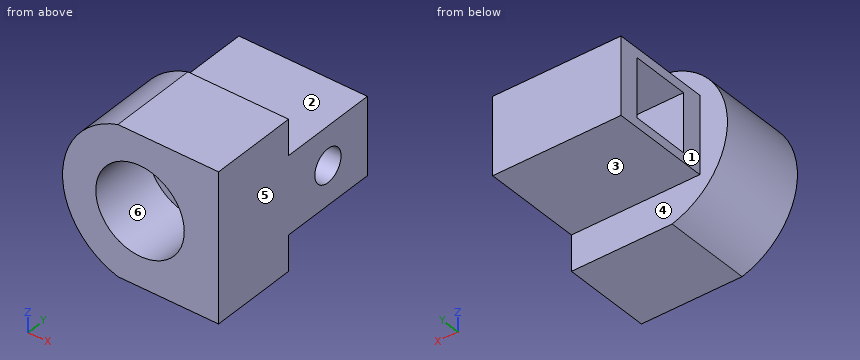
from build123d import *

# Parameters (mm, degrees)
SKETCH1_R           = 7
SKETCH1_R_2         = 4
BOSS_EXTRUDE1_DEPTH = 6
SKETCH2_R           = 7
BOSS_EXTRUDE2_DEPTH = 10
CUT_EXTRUDE1_DEPTH  = 8
SKETCH4_W           = 4.3
SKETCH4_H           = 6.3
CUT_EXTRUDE2_DEPTH  = 6
SKETCH5_OUTSIDE_W   = 21.092
SKETCH5_OUTSIDE_H   = 21.092
CUT_EXTRUDE3_DEPTH  = 8
BOSS_EXTRUDE3_DEPTH = 8
SKETCH9_R           = 7
CUT_EXTRUDE6_DEPTH  = 8
SKETCH10_W          = 9
SKETCH10_H          = 7
BOSS_EXTRUDE5_DEPTH = 9
SKETCH11_W          = 5.3
SKETCH11_H          = 5.3
CUT_EXTRUDE7_DEPTH  = 6
BOSS_EXTRUDE6_DEPTH = 8
SKETCH14_W          = 7
SKETCH14_H          = 9
BOSS_EXTRUDE7_DEPTH = 2.6
SKETCH15_W          = 4
SKETCH15_H          = 5
CUT_EXTRUDE10_DEPTH = 9
SKETCH16_R          = 1.5
CUT_EXTRUDE11_DEPTH = 6.6


with BuildPart() as part:
    # Sketch1 → Boss-Extrude1 (new body)
    with BuildSketch(Plane(origin=(0, 0, 0), x_dir=(1, 0, 0), z_dir=(0, 1, 0))):
        with Locations(Location((0, 0, 0), (0, 0, 270))):  # turned: the seam where the file's is
            Circle(SKETCH1_R)
        with Locations(Location((0, 0, 0), (0, 0, 270))):  # turned: the seam where the file's is
            Circle(SKETCH1_R_2, mode=Mode.SUBTRACT)
    extrude(amount=BOSS_EXTRUDE1_DEPTH)

    # Sketch2 → Boss-Extrude2 (add)
    with BuildSketch(Plane(origin=(0, 6, 0), x_dir=(1, 0, 0), z_dir=(0, 1, 0))):
        with Locations(Location((0, 0, 0), (0, 0, 270))):  # turned: the seam where the file's is
            Circle(SKETCH2_R)
    extrude(amount=BOSS_EXTRUDE2_DEPTH)

    # Sketch3 → Cut-Extrude1 (cut)
    with BuildSketch(Plane(origin=(0, 16, 0), x_dir=(1, 0, 0), z_dir=(0, 1, 0))):
        with BuildLine():
            Line((0, 7), (0, -7))
            ThreePointArc((0, -7), (-7, 0), (0, 7))
        make_face()
    extrude(amount=-CUT_EXTRUDE1_DEPTH, mode=Mode.SUBTRACT)

    # Sketch4 → Cut-Extrude2 (cut)
    with BuildSketch(Plane.ZY):
        with Locations((0, 12.15)):
            Rectangle(SKETCH4_W, SKETCH4_H)
    extrude(amount=-CUT_EXTRUDE2_DEPTH, mode=Mode.SUBTRACT)

    # Sketch5 outside → Cut-Extrude3 (cut)
    with BuildSketch(Plane(origin=(0, 16, 0), x_dir=(1, 0, 0), z_dir=(0, 1, 0))):
        Rectangle(SKETCH5_OUTSIDE_W, SKETCH5_OUTSIDE_H)
        with BuildLine():
            Line((0, 4), (5.744562647, 4))
            ThreePointArc((5.744562647, 4), (7, 0), (5.744562647, -4))
            Line((5.744562647, -4), (0, -4))
            Line((0, -4), (0, 4))
        make_face(mode=Mode.SUBTRACT)
    extrude(amount=-CUT_EXTRUDE3_DEPTH, mode=Mode.SUBTRACT)

    # Sketch7 → Boss-Extrude3 (add)
    with BuildSketch(Plane(origin=(0, 8, 0), x_dir=(1, 0, 0), z_dir=(0, 1, 0))):
        with BuildLine():
            Line((2, 6.708203932), (2, 11.708203932))
            Line((2, 11.708203932), (-2, 11.708203932))
            Line((-2, 11.708203932), (-2, 6.708203932))
            ThreePointArc((-2, 6.708203932), (0, 7), (2, 6.708203932))
        make_face()
        with BuildLine():
            Line((2, -6.708203932), (2, -11.708203932))
            Line((2, -11.708203932), (-2, -11.708203932))
            Line((-2, -11.708203932), (-2, -6.708203932))
            ThreePointArc((-2, -6.708203932), (0, -7), (2, -6.708203932))
        make_face()
    extrude(amount=-BOSS_EXTRUDE3_DEPTH)

    # Sketch9 → Cut-Extrude6 (cut)
    with BuildSketch(Plane(origin=(0, 16, 0), x_dir=(1, 0, 0), z_dir=(0, 1, 0))):
        Circle(SKETCH9_R)
    extrude(amount=-CUT_EXTRUDE6_DEPTH, mode=Mode.SUBTRACT)

    # Sketch10 → Boss-Extrude5 (add)
    with BuildSketch(Plane(origin=(0, 8, 0), x_dir=(1, 0, 0), z_dir=(0, 1, 0))):
        Rectangle(SKETCH10_W, SKETCH10_H)
    extrude(amount=BOSS_EXTRUDE5_DEPTH)

    # Sketch11 → Cut-Extrude7 (cut)
    with BuildSketch(Plane.ZY.offset(4.5)):
        with Locations((0, 12.5)):
            Rectangle(SKETCH11_W, SKETCH11_H)
    extrude(amount=-CUT_EXTRUDE7_DEPTH, mode=Mode.SUBTRACT)

    # Sketch13 → Boss-Extrude6 (add)
    with BuildSketch(Plane(origin=(0, 8, 0), x_dir=(1, 0, 0), z_dir=(0, 1, 0))):
        with BuildLine():
            Line((2, -6.708203932), (7.1, -6.708203932))
            Line((7.1, -6.708203932), (7.1, 6.708203932))
            Line((7.1, 6.708203932), (2, 6.708203932))
            ThreePointArc((2, 6.708203932), (7, 0), (2, -6.708203932))
        make_face()
    extrude(amount=-BOSS_EXTRUDE6_DEPTH)

    # Sketch14 → Boss-Extrude7 (add)
    with BuildSketch(Plane(origin=(4.5, 0, 0), x_dir=(0, 0, -1), z_dir=(1, 0, 0))):
        with Locations((0, 12.5)):
            Rectangle(SKETCH14_W, SKETCH14_H)
    extrude(amount=BOSS_EXTRUDE7_DEPTH)

    # Sketch15 → Cut-Extrude10 (cut, through all)
    with BuildSketch(Plane(origin=(0, 8, 0), x_dir=(1, 0, 0), z_dir=(0, 1, 0))):
        with Locations((0, 9.208203932)):
            Rectangle(SKETCH15_W, SKETCH15_H)
        with Locations((0, -9.208203932)):
            Rectangle(SKETCH15_W, SKETCH15_H)
    extrude(amount=-CUT_EXTRUDE10_DEPTH, mode=Mode.SUBTRACT)

    # Sketch16 → Cut-Extrude11 (cut, through all)
    with BuildSketch(Plane.ZY.offset(-1.5)):
        with Locations((0, 12.5)):
            Circle(SKETCH16_R)
    extrude(amount=-CUT_EXTRUDE11_DEPTH, mode=Mode.SUBTRACT)


solid = part.part
Build history of the part. All positions in model axes, mm. Face numbers are marked on the shaded views. A direction names the side the tool comes from. Round coordinates to 2 decimals unless told otherwise and drop trailing zeros. Loops run counter-clockwise (first coordinate to the right, second up) from the corner with the lowest first, then second, coordinate; pieces in that order, holes last. Notation, with made-up numbers: (-38.5, 27.5) -> (-16.5, 27.5) arc R10 ccw to (-16.5, 35.5) -> close; hole circle Ø8 at (8.25, 33.5). An arc over 180 degrees is marked (long way). One line per item, written item: value. Start each with the question number.
Q1. 3-axis set-ups, long thin cutter, end or side, ignore diameter. For the marked faces 1, 2 and 3: which of +Z, -Z, +X, -X, +Y, -Y reach the whole face in a straight line?
Q2. Cut at B-B on x = 0. List the corners of the cut face in (y, z).
Q3. Two-plate mould, pull along X, no slides. Class the marked faces 4, 5 and 6: released by +X, released by -X, zero draft, split by the parting line, or undercut.
Q4. Probe line 1 along Z through (x, y) = (-2.25, 14); line 2 along Y through (x, z) = (4.75, -4.5); line 3 along X through (y, z) = (7.75, 2). List the from-to ranges inside material, lowest first.
Q5. Drop flat-ended pins along their axis: pin 1 Ø1 at (y, z) = (4.5, 0.5) entering from -X; pin 2 Ø7.5 at (y, z) = (14, 1.5) entering from -X; pin 3 Ø7 at (x, y) = (1, 12) entering from -Z; pin 4 Ø6 at (x, y) = (-2, 12.5) entering from +Z. Give the stop position or say it passes through.
Q6. Cut at C-C on z = 0.25. List the corners of the cut face in (x, y).
Q7. Cut at A-A on y = 12.5. List the corners of the cut face in (x, z), plus the area to 3 significant figures.
Q8. Cut at D-D on y = 1.25. List the corners of the cut face in (x, z), plus the area to 3 significant figures.
Computed:
1. face 1: +Z, -Z, -X, +Y
1. face 2: +Z, +X, -X, +Y
1. face 3: -Z, +X, -X, +Y
2. outline: (0, -6.71) -> (8, -6.71) -> (8, -3.5) -> (17, -3.5) -> (17, 3.5) -> (8, 3.5) -> (8, 6.71) -> (0, 6.71) -> (0, 4) -> (6, 4) -> (6, -4) -> (0, -4) -> close; hole (9.85, -2.65) -> (15.15, -2.65) -> (15.15, 2.65) -> (9.85, 2.65) -> close
3. face 4: zero draft
3. face 5: released by +X
3. face 6: undercut
4. line 1: -3.5 to -2.65, 2.65 to 3.5
4. line 2: 0 to 8
4. line 3: -6.71 to 7.1
5. pin 1: x = -7
5. pin 2: x = -4.5
5. pin 3: z = -3.5
5. pin 4: z = 3.5
6. outline: (-7, 0) -> (-3.99, 0) -> (-3.99, 6) -> (3.99, 6) -> (3.99, 0) -> (7.1, 0) -> (7.1, 11.02) -> (1.5, 11.02) -> (1.5, 9.85) -> (-4.5, 9.85) -> (-4.5, 8) -> (-7, 8) -> close; (-4.5, 15.15) -> (1.5, 15.15) -> (1.5, 13.98) -> (7.1, 13.98) -> (7.1, 17) -> (-4.5, 17) -> close
7. outline: (-4.5, -3.5) -> (7.1, -3.5) -> (7.1, -1.5) -> (1.5, -1.5) -> (1.5, -2.65) -> (-4.5, -2.65) -> close; (-4.5, 2.65) -> (1.5, 2.65) -> (1.5, 1.5) -> (7.1, 1.5) -> (7.1, 3.5) -> (-4.5, 3.5) -> close
7. area: 32.6 mm²
8. outline: (-2, -6.71) -> (7.1, -6.71) -> (7.1, 6.71) -> (-2, 6.71) arc R7 ccw to start; hole circle Ø8 at (0, 0)
8. area: 121 mm²
